Source: CAD feature listing. Evaluate the final solid. Frame: model axes, mm. Face numbers are marked on the shaded views. A direction names the side the tool comes from. Round coordinates to 2 decimals unless told otherwise and drop trailing zeros. Loops run counter-clockwise (first coordinate to the right, second up) from the corner with the lowest first, then second, coordinate; pieces in that order, holes last.
(1) Section B-B, the plane z = 18.5. Return the cut outline in (x, y), plus the area to 3 significant figures.
(2) Set-up query: the marked faces 1, 2 and 3. Return all of +Z, -Z, +X, -X, +Y, -Y with unobstructed straight access to the full face (end or side cutting, diameter ignored); none if empty.
(3) Material intervals for probe 1 along Z at (x, y) = (-8.75, 0.25); probe 2 along X at (y, z) = (0.5, 27.5); probe 3 along Z at (x, y) = (-2.5, -4), sorted ascending.
(4) Section C-C, the plane z = 52.5. Return the cut outline in (x, y), plus the area to 3 significant figures.
(5) First-contact query: pin 1 Ø1.3 at (x, y) = (-6.5, 3.5) entering from -Z; pin 2 Ø3 at (x, y) = (7.51, -7.51) entering from +Z; pin 3 Ø12 at (x, z) = (6, 49) entering from +Y. Flat tips, straight axial feed; report the tip coordinate or a pass-through.
```python
from build123d import *
from OCP.BRepFilletAPI import BRepFilletAPI_MakeChamfer

# Parameters (mm, degrees)
SKETCH1_R         = 11
EXTRUDE1_DEPTH    = 47
SKETCH2_R         = 10.75
EXTRUDE2_DEPTH    = 1
EXTRUDE3_START    = 0.5
SKETCH3_R         = 10.75
EXTRUDE3_DEPTH    = 0.5
SKETCH4_R         = 5
EXTRUDE4_DEPTH    = 1
EXTRUDE5_START    = 1
SKETCH5_R         = 5
EXTRUDE5_DEPTH    = 1
SKETCH6_R         = 1.5
EXTRUDE6_DEPTH    = 10
EXTRUDE7_START    = 6.5
SKETCH7_R         = 1.5
EXTRUDE7_DEPTH    = 6.5
CHAMFER1_SIZE     = 0.75
CHAMFER1_SIZE2    = 0.433012702
SKETCH8_R         = 1
EXTRUDE8_DEPTH    = 3
CIRPATTERN1_COUNT = 3
SKETCH9_R         = 0.8
EXTRUDE9_DEPTH    = 2.4
CIRPATTERN2_COUNT = 3
EXTRUDE10_START   = -1
EXTRUDE10_DEPTH   = 1
CIRPATTERN3_COUNT = 4


with BuildPart() as part:
    # Sketch1 → Extrude1 (new body)
    with BuildSketch(Plane.XY):
        Circle(SKETCH1_R)
    extrude(amount=EXTRUDE1_DEPTH)

    # Sketch2 → Extrude2 (add)
    with BuildSketch(Plane.XY.offset(47)):
        Circle(SKETCH2_R)
    extrude(amount=EXTRUDE2_DEPTH)

    # Sketch3 → Extrude3 (add)
    with BuildSketch(Plane(origin=(0, 0, 0), x_dir=(-1, 0, 0), z_dir=(0, 0, -1)).offset(EXTRUDE3_START)):
        with Locations(Location((0, 0, 0), (0, 0, 180))):
            Circle(SKETCH3_R)
    extrude(amount=-EXTRUDE3_DEPTH)

    # Sketch4 → Extrude4 (add)
    with BuildSketch(Plane.XY.offset(48)):
        Circle(SKETCH4_R)
    extrude(amount=EXTRUDE4_DEPTH)

    # Sketch5 → Extrude5 (add)
    with BuildSketch(Plane(origin=(0, 0, -0.5), x_dir=(-1, 0, 0), z_dir=(0, 0, -1)).offset(EXTRUDE5_START)):
        with Locations(Location((0, 0, 0), (0, 0, 180))):
            Circle(SKETCH5_R)
    extrude(amount=-EXTRUDE5_DEPTH)

    # Sketch6 → Extrude6 (add)
    with BuildSketch(Plane.XY.offset(49)):
        Circle(SKETCH6_R)
    extrude(amount=EXTRUDE6_DEPTH)

    # Sketch7 → Extrude7 (add)
    with BuildSketch(Plane(origin=(0, 0, -1.5), x_dir=(-1, 0, 0), z_dir=(0, 0, -1)).offset(EXTRUDE7_START)):
        with Locations(Location((0, 0, 0), (0, 0, 180))):
            Circle(SKETCH7_R)
    extrude(amount=-EXTRUDE7_DEPTH)

    # Chamfer1: one chamfer whose edges measure the first distance from different faces: ONE call of the kernel's chamfer builder (chamfer() names one face for all edges)
    chamfer1_edges_1 = [part.edges().sort_by_distance(p)[0] for p in [
        (-1.5, 0, 59),
    ]]
    chamfer1_side_1 = [part.faces().sort_by_distance(p)[0] for p in [
        (-1.5, 0, 54),
    ]]
    chamfer1_edges_2 = [part.edges().sort_by_distance(p)[0] for p in [
        (-1.5, 0, -8),
    ]]
    chamfer1_side_2 = [part.faces().sort_by_distance(p)[0] for p in [
        (-1.5, 0, -4.75),
    ]]
    chamfer1 = BRepFilletAPI_MakeChamfer(part.part.solid().wrapped)
    for e in chamfer1_edges_1:
        chamfer1.Add(CHAMFER1_SIZE, CHAMFER1_SIZE2, e.wrapped, chamfer1_side_1[0].wrapped)  # the first distance lies on this face
    for e in chamfer1_edges_2:
        chamfer1.Add(CHAMFER1_SIZE, CHAMFER1_SIZE2, e.wrapped, chamfer1_side_2[0].wrapped)  # the first distance lies on this face
    add(Compound.cast(chamfer1.Shape()), mode=Mode.REPLACE)

    # Sketch8 → Extrude8 (cut)
    with BuildSketch(Plane.XY.offset(48)):
        with Locations((0, -8.5)):
            Circle(SKETCH8_R)
    extrude8 = extrude(amount=-EXTRUDE8_DEPTH, mode=Mode.SUBTRACT)

    # CirPattern1: Extrude8 ×3 about axis
    cirpattern1_axis = Axis((0, 0, 0), (0, 0, 1))
    for i in range(1, CIRPATTERN1_COUNT):
        add(extrude8.rotate(cirpattern1_axis, i * 360 / CIRPATTERN1_COUNT), mode=Mode.SUBTRACT)

    # Sketch9 → Extrude9 (cut)
    with BuildSketch(Plane(origin=(0, 0, -0.5), x_dir=(-1, 0, 0), z_dir=(0, 0, -1))):
        with Locations((0, -7.5)):
            Circle(SKETCH9_R)
    extrude9 = extrude(amount=-EXTRUDE9_DEPTH, mode=Mode.SUBTRACT)

    # CirPattern2: Extrude9 ×3 about axis
    cirpattern2_axis = Axis((0, 0, 0), (0, 0, 1))
    for i in range(1, CIRPATTERN2_COUNT):
        add(extrude9.rotate(cirpattern2_axis, i * 360 / CIRPATTERN2_COUNT), mode=Mode.SUBTRACT)

    # Sketch11 → Extrude10 (cut)
    with BuildSketch(Plane.XY.offset(48).offset(EXTRUDE10_START)):
        with BuildLine():
            ThreePointArc((6.864194516, 8.273169505), (6.800769225, 6.800769225), (8.273169505, 6.864194516))
            ThreePointArc((8.273169505, 6.864194516), (7.601397898, 7.601397898), (6.864194516, 8.273169505))
        make_face()
    extrude10 = extrude(amount=EXTRUDE10_DEPTH, mode=Mode.SUBTRACT)

    # CirPattern3: Extrude10 ×4 about axis
    cirpattern3_axis = Axis((0, 0, 0), (0, 0, 1))
    for i in range(1, CIRPATTERN3_COUNT):
        add(extrude10.rotate(cirpattern3_axis, i * 360 / CIRPATTERN3_COUNT), mode=Mode.SUBTRACT)


solid = part.part
```
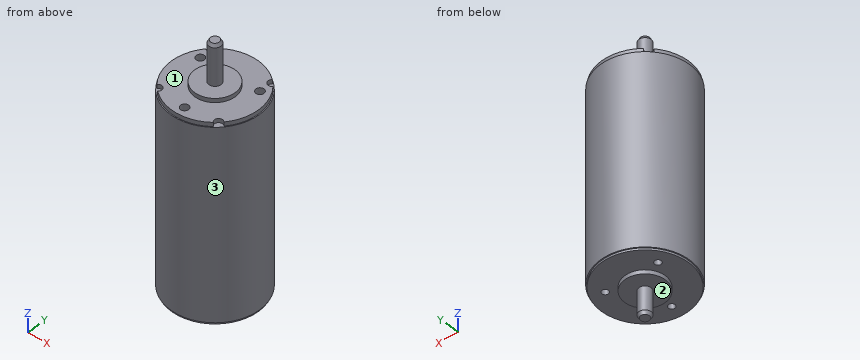
Output values:
1. outline: circle Ø22 at (0, 0)
1. area: 380 mm2
2. face 1: +Z
2. face 2: -Z
2. face 3: +Z, -Z
3. probe 1: z = -0.5 to 48
3. probe 2: x = -10.99 to 10.99
3. probe 3: z = -1.5 to 49
4. outline: circle Ø3 at (0, 0)
4. area: 7.07 mm2
5. pin 1: stops at z = -0.5
5. pin 2: stops at z = 48
5. pin 3: stops at y = 10.99
